Source: CAD feature listing. Evaluate the final solid. Frame: model axes, mm. A direction names the side the tool comes from. Give positions to 0.01 mm unless a question says otherwise; leave off trailing zeros. Write each loop counter-clockwise with the first axis right and the second up, starting at its lowest first coordinate (ties: lowest second). Pieces come first, ordered by that corner, then holes. Notation, with made-up numbers: M 73.25,45.25 L 103.25,45.25 A21 ccw 103.25,51.25 Z; hole C 73,33 d4. An arc over 180 degrees is marked long. Answer as a JSON object with one key per item and string values. Group by question number.
```python
from build123d import *

# Parameters (mm, degrees)
SKETCH1_W            = 10
SKETCH1_H            = 26
BOSS_EXTRUDE1_DEPTH  = 1
BOSS_EXTRUDE5_DEPTH  = 3.6
SKETCH6_W            = 1.45
SKETCH6_H            = 2.6
BOSS_EXTRUDE9_DEPTH  = 26
SKETCH7_W            = 0.55
SKETCH7_H            = 1.7
CUT_EXTRUDE1_DEPTH   = 26
CUT_EXTRUDE3_DEPTH   = 0.9
CUT_EXTRUDE4_DEPTH   = 1.7
FILLET1_R            = 0.25
FILLET2_R            = 1
SKETCH12_R           = 0.75
BOSS_EXTRUDE10_DEPTH = 5


with BuildPart() as part:
    # Sketch1 → Boss-Extrude1 (new body)
    with BuildSketch(Plane.XY):
        with Locations((5, 13)):
            Rectangle(SKETCH1_W, SKETCH1_H)
    extrude(amount=BOSS_EXTRUDE1_DEPTH)

    # Sketch2 → Boss-Extrude5 (add)
    with BuildSketch(Plane(origin=(0, 0, 0), x_dir=(-1, 0, 0), z_dir=(0, 0, -1))):
        with BuildLine():
            Line((-10, 26), (0, 26))
            ThreePointArc((0, 26), (-5, 31), (-10, 26))
        make_face()
    extrude(amount=-BOSS_EXTRUDE5_DEPTH)

    # Sketch6 → Boss-Extrude9 (add)
    with BuildSketch(Plane.XZ):
        with Locations((0.725, 2.3)):
            Rectangle(SKETCH6_W, SKETCH6_H)
        with Locations((9.275, 2.3)):
            Rectangle(SKETCH6_W, SKETCH6_H)
    extrude(amount=-BOSS_EXTRUDE9_DEPTH)

    # Sketch7 → Cut-Extrude1 (cut)
    with BuildSketch(Plane.XZ):
        with Locations((1.175, 1.85)):
            Rectangle(SKETCH7_W, SKETCH7_H)
        with Locations((8.825, 1.85)):
            Rectangle(SKETCH7_W, SKETCH7_H)
    extrude(amount=-CUT_EXTRUDE1_DEPTH, mode=Mode.SUBTRACT)

    # Sketch10 → Cut-Extrude3 (cut)
    with BuildSketch(Plane.XY.offset(3.6)):
        with BuildLine():
            Line((1.45, 26), (8.55, 26))
            ThreePointArc((8.55, 26), (5, 29.55), (1.45, 26))
        make_face()
    extrude(amount=-CUT_EXTRUDE3_DEPTH, mode=Mode.SUBTRACT)

    # Sketch11 → Cut-Extrude4 (cut)
    with BuildSketch(Plane.XY.offset(1)):
        with BuildLine():
            Line((0.9, 26), (9.1, 26))
            ThreePointArc((9.1, 26), (5, 30.1), (0.9, 26))
        make_face()
    extrude(amount=CUT_EXTRUDE4_DEPTH, mode=Mode.SUBTRACT)

    # Fillet1
    fillet1_edges = [part.edges().sort_by_distance(p)[0] for p in [
        (1.45, 13, 3.6),
        (8.55, 13, 3.6),
        (1.45, 13, 2.7),
        (8.55, 13, 2.7),
        (5, 29.55, 2.7),
        (5, 29.55, 3.6),
    ]]
    fillet(fillet1_edges, radius=FILLET1_R)

    # Fillet2
    fillet2_edges = [part.edges().sort_by_distance(p)[0] for p in [
        (5, 31, 0),
        (10, 13, 0),
        (0, 13, 0),
    ]]
    fillet(fillet2_edges, radius=FILLET2_R)

    # Sketch12 → Boss-Extrude10 (add)
    with BuildSketch(Plane(origin=(0, 0, 0), x_dir=(-1, 0, 0), z_dir=(0, 0, -1))):
        with Locations((-5, 4)):
            Circle(SKETCH12_R)
    extrude(amount=BOSS_EXTRUDE10_DEPTH)


solid = part.part
```
(1) Pull-direction query (X, two-part tool) for faces 4 (the cylindrical face through (5, 31, 2)), 5 (the cylindrical face through (0.285, 13.182, 0.301)), 6 (the cylindrical face through (5.08, 29.55, 3.15)); classes: pulls with the +X half, pulls with the -X half, needs draft (parallel to the pull), parting line crosses it, or undercut.
(2) Section C-C, the plane z = -1.75. Return loops of the section in (x, y), plus the area to 3 significant figures.
(3) Ray query, L1, parallel to X at y = 13, z = 1.5; L2, parallel to Z at x = 9, y = 10.5; L3, parallel to Z at x = 4.75, y = 11.5. Return the intervals inside material, ascending. Write a range as [from, to].
(4) Section A-A, the plane x = 5. Return loops of the section in (y, z), plus the area to 3 significant figures.
(5) Access query for faces 1 (the flat face through (0.9, 13, 2)), 2 (the cylindrical face through (5.595, 3.544, -2.465)), 3 (the cylindrical face through (9.715, 12.818, 0.301)). Directions: +Z, -Z, +X, -X, +Y, -Y. A direction counts if a zero-diameter tool reaches every point of the face in a straight line with its end or side. Return the directions, or none.
(6) Section B-B, the plane y = 5.5. Return loops of the section in (x, z), plus the area to 3 significant figures.
(7) Contact query for flat-ended pins moving along their axis: pin 1 Ø4 at (x, y) = (6, 16) entering from -Z; pin 2 Ø3 at (y, z) = (17, -1) entering from -X; pin 3 Ø6 at (x, y) = (5, 24.5) entering from +Z; pin 4 Ø1 at (x, z) = (1.5, -1.5) entering from +Y. Output: stop coordinate, or through.
Reported:
{
 "1": {"face 4": "parting line crosses it", "face 5": "pulls with the -X half", "face 6": "undercut"},
 "2": {"outline": "C 5,4 d1.5", "area": "1.77 mm2"},
 "3": {"L1": "x = [0, 0.9], [9.1, 10]", "L2": "z = [0, 1], [2.7, 3.6]", "L3": "z = [0, 1]"},
 "4": {"outline": "M 0,0 L 3.25,0 L 3.25,-5 L 4.75,-5 L 4.75,0 L 30,0 A1 ccw 31,1 L 31,3.6 L 29.8,3.6 A0.25 ccw 29.55,3.35 L 29.55,2.95 A0.25 ccw 29.8,2.7 L 30.1,2.7 L 30.1,1 L 0,1 Z", "area": "41.1 mm2"},
 "5": {"face 1": "-Y", "face 2": "-Z", "face 3": "-Z, +X, +Y, -Y"},
 "6": {"outline": "M 0,1 A1 ccw 1,0 L 9,0 A1 ccw 10,1 L 10,3.6 L 8.8,3.6 A0.25 ccw 8.55,3.35 L 8.55,2.95 A0.25 ccw 8.8,2.7 L 9.1,2.7 L 9.1,1 L 0.9,1 L 0.9,2.7 L 1.2,2.7 A0.25 ccw 1.45,2.95 L 1.45,3.35 A0.25 ccw 1.2,3.6 L 0,3.6 Z", "area": "15.2 mm2"},
 "7": {"pin 1": "stops at z = 0", "pin 2": "stops at x = 0.13", "pin 3": "stops at z = 1", "pin 4": "passes through"}
}
